Study the drawing (mm; zero at the part's minimum x, y, z) and answer. A direction names the side the tool comes from. Give positions to 0.01 mm unless a question says otherwise; leave off trailing zeros. Order: outer loops, then holes, each group sorted by start corner. A loop starts at its lowest first (then second) coordinate and runs counter-clockwise, first axis right, second up. Notation, with made-up numbers: (39.25, -22) - (45.25, -22) arc R16 ccw to (45.25, -13) - close; hole circle Ø9 at (59.25, 24). An arc over 180 degrees is marked (long way). Return JSON: item names as keys, results as strings.
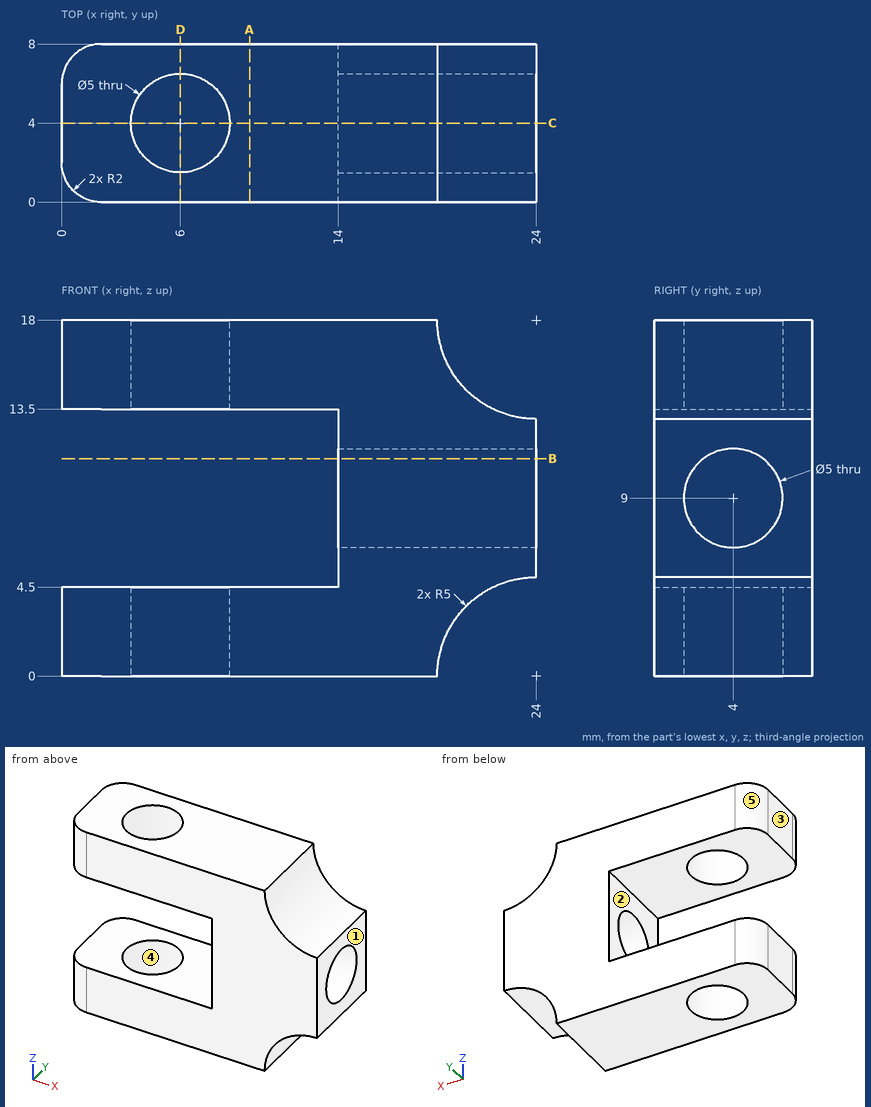
Q1. A cutting plane is placed at A-A (x = 9.5). Write down the section's boundary in (y, z), and give its area (3 significant figures).
Values:
{"outline": "(0, 0) - (8, 0) - (8, 4.5) - (0, 4.5) - close; (0, 13.5) - (8, 13.5) - (8, 18) - (0, 18) - close", "area": "72.0 mm²"}
Q2. A cutting plane is placed at D-D (x = 6). Write down the section's boundary in (y, z).
Values:
{"outline": "(0, 0) - (1.5, 0) - (1.5, 4.5) - (0, 4.5) - close; (0, 13.5) - (1.5, 13.5) - (1.5, 18) - (0, 18) - close; (6.5, 0) - (8, 0) - (8, 4.5) - (6.5, 4.5) - close; (6.5, 13.5) - (8, 13.5) - (8, 18) - (6.5, 18) - close"}
Q3. For the marked faces 1 and 2, determine the directions among +Z, -Z, +X, -X, +Y, -Y from which every point of the face is accessible in a straight line to the end or side of a thin tool.
Values:
{"face 1": "+Z, -Z, +X, +Y, -Y", "face 2": "-X, +Y, -Y"}
Q4. Determine the mould class of the marked faces 3, 4 and 5 for opening direction Y: released by +Y, released by -Y, zero draft, split by the parting line, or undercut.
Values:
{"face 3": "zero draft", "face 4": "undercut", "face 5": "released by +Y"}
Q5. A cutting plane is placed at B-B (z = 11). Write down the section's boundary in (x, y), and give its area (3 significant figures).
Values:
{"outline": "(14, 0) - (24, 0) - (24, 2.5) - (14, 2.5) - close; (14, 5.5) - (24, 5.5) - (24, 8) - (14, 8) - close", "area": "50.0 mm²"}
Q6. A cutting plane is placed at C-C (y = 4). Write down the section's boundary in (x, z), and give its area (3 significant figures).
Values:
{"outline": "(0, 0) - (3.5, 0) - (3.5, 4.5) - (0, 4.5) - close; (0, 13.5) - (3.5, 13.5) - (3.5, 18) - (0, 18) - close; (8.5, 0) - (19, 0) arc R5 cw to (24, 5) - (24, 6.5) - (14, 6.5) - (14, 4.5) - (8.5, 4.5) - close; (8.5, 13.5) - (14, 13.5) - (14, 11.5) - (24, 11.5) - (24, 13) arc R5 cw to (19, 18) - (8.5, 18) - close", "area": "172 mm²"}
Q7. Consider L1, parallel to Z at x = 3.5, y = 3; L2, parallel to Y at x = 6, z = 17; L3, parallel to X at y = 5.25, z = 2.5. Determine where each line is inside the solid, lowest interval first.
Values:
{"L1": "z = 0 to 4.5, 13.5 to 18", "L2": "y = 0 to 1.5, 6.5 to 8", "L3": "x = 0 to 3.83, 8.17 to 19.67"}
Q8. Given pin 1 (3 mm diameter, centred on y = 1, z = 8.5, fed in from -X); pin 2 (4.5 mm diameter, centred on y = 4, z = 9, fed in from +X); pin 3 (1 mm diameter, centred on x = 20, y = 1.5, fed in from -Z), each flat-ended and moving along its own axis, determine where each tip first touches the part or whether it passes through.
Values:
{"pin 1": "stops at x = 14", "pin 2": "passes through", "pin 3": "stops at z = 2.18"}
